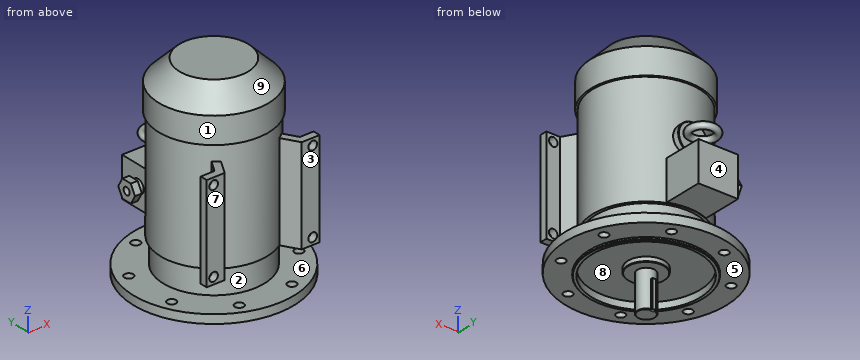
from build123d import *

# Parameters (mm, degrees)
SKETCH_1_R           = 19
EXTRUDE_1_DEPTH      = 80
SKETCH_2_W           = 8
SKETCH_2_H           = 8
EXTRUDE_2_DEPTH      = 0.1
EXTRUDE_2_DEPTH_BACK = 60
SKETCH_3_R           = 175
EXTRUDE_3_DEPTH      = 19
SKETCH_4_R           = 125
SKETCH_4_R_2         = 118
EXTRUDE_4_DEPTH      = 5
SKETCH_5_R           = 118
SKETCH_5_R_2         = 40
CUT_EXTRUDE_1_DEPTH  = 10
CHAMFER_1_SIZE       = 1
SKETCH_6_R           = 9.5
CUT_EXTRUDE_2_DEPTH  = 20
SKETCH_7_R           = 110
EXTRUDE_5_DEPTH      = 55
SKETCH_8_R           = 116
EXTRUDE_6_DEPTH      = 242
SKETCH_9_R           = 120
EXTRUDE_7_DEPTH      = 102
CHAMFER_2_SIZE       = 45
EXTRUDE_8_DEPTH      = 208
CUT_EXTRUDE_3_REACH  = 309
SKETCH_11_R          = 9.5
SKETCH_12_W          = 86
SKETCH_12_H          = 86
EXTRUDE_9_DEPTH      = 193
SKETCH_13_R          = 32
EXTRUDE_10_DEPTH     = 126
CHAMFER_3_SIZE       = 1
SKETCH_15_R          = 7
SKETCH_16_R          = 15
EXTRUDE_11_DEPTH     = 10
EXTRUDE_12_DEPTH     = 15
SKETCH_18_R          = 8
CUT_EXTRUDE_4_DEPTH  = 15


with BuildPart() as part:
    # Эскиз1 → Вытянуть1 (new body)
    with BuildSketch(Plane.XY):
        Circle(SKETCH_1_R)
    extrude(amount=EXTRUDE_1_DEPTH)

    # Эскиз2 → Вытянуть2 (add, two sides)
    with BuildSketch(Plane(origin=(0, 0, 0), x_dir=(-1, 0, 0), z_dir=(0, 0, -1))) as extrude_2_sk:
        with Locations((0, 18)):
            Rectangle(SKETCH_2_W, SKETCH_2_H)
    extrude(amount=EXTRUDE_2_DEPTH)
    extrude(extrude_2_sk.sketch, amount=-EXTRUDE_2_DEPTH_BACK)

    # Эскиз3 → Вытянуть3 (add)
    with BuildSketch(Plane.XY.offset(80)):
        Circle(SKETCH_3_R)
    extrude(amount=EXTRUDE_3_DEPTH)

    # Эскиз4 → Вытянуть4 (add)
    with BuildSketch(Plane(origin=(0, 0, 80), x_dir=(-1, 0, 0), z_dir=(0, 0, -1))):
        with Locations(Location((0, 0, 0), (0, 0, 180))):  # turned: the seam where the file's is
            Circle(SKETCH_4_R)
        Circle(SKETCH_4_R_2, mode=Mode.SUBTRACT)
    extrude(amount=EXTRUDE_4_DEPTH)

    # Эскиз5 → Вырез-Вытянуть1 (cut)
    with BuildSketch(Plane(origin=(0, 0, 80), x_dir=(-1, 0, 0), z_dir=(0, 0, -1))):
        Circle(SKETCH_5_R)
        Circle(SKETCH_5_R_2, mode=Mode.SUBTRACT)
    extrude(amount=-CUT_EXTRUDE_1_DEPTH, mode=Mode.SUBTRACT)

    # Фаска1
    chamfer_1_edges = [part.edges().sort_by_distance(p)[0] for p in [
        (-125, 0, 75),
        (40, 0, 80),
        (-11.937336386, -14.781745499, 0),
    ]]
    chamfer(chamfer_1_edges, length=CHAMFER_1_SIZE)

    # Эскиз6 → Вырез-Вытянуть2 (cut, through all)
    with BuildSketch(Plane(origin=(0, 0, 80), x_dir=(-1, 0, 0), z_dir=(0, 0, -1))):
        with Locations((-57.402514855, 138.581929877)):
            Circle(SKETCH_6_R)
        with Locations((57.402514855, 138.581929877)):
            Circle(SKETCH_6_R)
        with Locations((138.581929877, 57.402514855)):
            Circle(SKETCH_6_R)
        with Locations((138.581929877, -57.402514855)):
            Circle(SKETCH_6_R)
        with Locations((57.402514855, -138.581929877)):
            Circle(SKETCH_6_R)
        with Locations((-57.402514855, -138.581929877)):
            Circle(SKETCH_6_R)
        with Locations((-138.581929877, -57.402514855)):
            Circle(SKETCH_6_R)
        with Locations((-138.581929877, 57.402514855)):
            Circle(SKETCH_6_R)
    extrude(amount=-CUT_EXTRUDE_2_DEPTH, mode=Mode.SUBTRACT)

    # Эскиз7 → Вытянуть5 (add)
    with BuildSketch(Plane.XY.offset(99)):
        Circle(SKETCH_7_R)
    extrude(amount=EXTRUDE_5_DEPTH)

    # Эскиз8 → Вытянуть6 (add)
    with BuildSketch(Plane.XY.offset(154)):
        Circle(SKETCH_8_R)
    extrude(amount=EXTRUDE_6_DEPTH)

    # Эскиз9 → Вытянуть7 (add)
    with BuildSketch(Plane.XY.offset(396)):
        Circle(SKETCH_9_R)
    extrude(amount=EXTRUDE_7_DEPTH)

    # Фаска2
    chamfer_2_edges = [part.edges().sort_by_distance(p)[0] for p in [
        (-120, 0, 498),
    ]]
    chamfer(chamfer_2_edges, length=CHAMFER_2_SIZE)

    # Эскиз10 → Вытянуть8 (add)
    with BuildSketch(Plane(origin=(0, 0, 154), x_dir=(-1, 0, 0), z_dir=(0, 0, -1))):
        Polygon((-123, -132), (-83.762395693, -132), (-58.16412012, -87.662486121), (-72.020526581, -79.662486121), (-93, -116), (-123, -116), align=None)
        Polygon((123, -132), (83.762395693, -132), (58.16412012, -87.662486121), (72.020526581, -79.662486121), (93, -116), (123, -116), align=None)
    extrude(amount=-EXTRUDE_8_DEPTH)

    # Эскиз11 → Вырез-Вытянуть3 (cut, up to next)
    with BuildSketch(Plane.XZ.offset(132), mode=Mode.PRIVATE) as cut_extrude_3_sk1:
        with Locations((-108, 169)):
            Circle(SKETCH_11_R)
    cut_extrude_3_tool1 = extrude(cut_extrude_3_sk1.sketch, amount=-CUT_EXTRUDE_3_REACH, mode=Mode.PRIVATE) & part.part
    add(cut_extrude_3_tool1.solids().sort_by_distance((-108, -132, 169))[0], mode=Mode.SUBTRACT)
    # Эскиз11 → Вырез-Вытянуть3 (cut, up to next)
    with BuildSketch(Plane.XZ.offset(132), mode=Mode.PRIVATE) as cut_extrude_3_sk2:
        with Locations((108, 169)):
            Circle(SKETCH_11_R)
    cut_extrude_3_tool2 = extrude(cut_extrude_3_sk2.sketch, amount=-CUT_EXTRUDE_3_REACH, mode=Mode.PRIVATE) & part.part
    add(cut_extrude_3_tool2.solids().sort_by_distance((108, -132, 169))[0], mode=Mode.SUBTRACT)
    # Эскиз11 → Вырез-Вытянуть3 (cut, up to next)
    with BuildSketch(Plane.XZ.offset(132), mode=Mode.PRIVATE) as cut_extrude_3_sk3:
        with Locations((-108, 347)):
            Circle(SKETCH_11_R)
    cut_extrude_3_tool3 = extrude(cut_extrude_3_sk3.sketch, amount=-CUT_EXTRUDE_3_REACH, mode=Mode.PRIVATE) & part.part
    add(cut_extrude_3_tool3.solids().sort_by_distance((-108, -132, 347))[0], mode=Mode.SUBTRACT)
    # Эскиз11 → Вырез-Вытянуть3 (cut, up to next)
    with BuildSketch(Plane.XZ.offset(132), mode=Mode.PRIVATE) as cut_extrude_3_sk4:
        with Locations((108, 347)):
            Circle(SKETCH_11_R)
    cut_extrude_3_tool4 = extrude(cut_extrude_3_sk4.sketch, amount=-CUT_EXTRUDE_3_REACH, mode=Mode.PRIVATE) & part.part
    add(cut_extrude_3_tool4.solids().sort_by_distance((108, -132, 347))[0], mode=Mode.SUBTRACT)

    # Эскиз12 → Вытянуть9 (add)
    with BuildSketch(Plane(origin=(0, 0, 0), x_dir=(1, 0, 0), z_dir=(0, 1, 0))):
        with Locations((0, -198)):
            Rectangle(SKETCH_12_W, SKETCH_12_H)
    extrude(amount=EXTRUDE_9_DEPTH)

    # Эскиз13 → Вытянуть10 (add)
    with BuildSketch(Plane(origin=(0, 0, 0), x_dir=(1, 0, 0), z_dir=(0, 1, 0))):
        with Locations(Location((0, -286, 0), (0, 0, 90))):  # turned: the seam where the file's is
            Circle(SKETCH_13_R)
    extrude(amount=EXTRUDE_10_DEPTH)

    # Фаска3
    chamfer_3_edges = [part.edges().sort_by_distance(p)[0] for p in [
        (0, 126, 318),
    ]]
    chamfer(chamfer_3_edges, length=CHAMFER_3_SIZE)

    # По траектории1: sweep along a path in Эскиз14
    with BuildLine(Plane.XY.offset(286)) as sweep_1_path:
        CenterArc((0, 152), 26, 0, 360)
    # Эскиз15 → По траектории1 (sweep)
    with BuildSketch(Plane(origin=(0, 0, 0), x_dir=(0, 0, -1), z_dir=(1, 0, 0))):
        with Locations((-286, 178)):
            Circle(SKETCH_15_R)
    sweep(path=sweep_1_path.line)

    # Эскиз16 → Вытянуть11 (add)
    with BuildSketch(Plane.ZY.offset(43)):
        with Locations(Location((198, 150, 0), (0, 0, 180))):  # turned: the seam where the file's is
            Circle(SKETCH_16_R)
    extrude(amount=EXTRUDE_11_DEPTH)

    # Эскиз17 → Вытянуть12 (add)
    with BuildSketch(Plane.ZY.offset(53)):
        Polygon((198, 172.516660498), (178.5, 161.258330249), (178.5, 138.741669751), (198, 127.483339502), (217.5, 138.741669751), (217.5, 161.258330249), align=None)
    extrude(amount=EXTRUDE_12_DEPTH)

    # Эскиз18 → Вырез-Вытянуть4 (cut)
    with BuildSketch(Plane.ZY.offset(68)):
        with Locations((198, 150)):
            Circle(SKETCH_18_R)
    extrude(amount=-CUT_EXTRUDE_4_DEPTH, mode=Mode.SUBTRACT)


solid = part.part
Geometry check sheet. Reference: the model listing, model coordinates, mm. Face numbers are marked on the shaded views. A direction names the side the tool comes from. Coordinates: 2 decimals unless noted, no trailing zeros. Order: outer loops, then holes, each group sorted by start corner. A loop starts at its lowest first (then second) coordinate and runs counter-clockwise, first axis right, second up. Notation, with made-up numbers: (59, 1.25) - (74, 1.25) arc R23 ccw to (74, 39.25) - close; hole circle Ø4 at (4.25, -26.75). An arc over 180 degrees is marked (long way). Answer in a Markdown table with one row per item. Add a question column.
1) Release check for a two-part mould opening along Z. For the marked faces 6, 7, 8 and 9 record: +Z half, -Z half, draft (parallel to the pull), parting line (faces both ways), or undercut.
2) Cross-section at A-A, the plane z = 347. Record the cut outline in (x, y).
3) Gauge pin test, flat ends, axial feed: P1, Ø9, axis at y = 18.5, z = 37, coming from the -X side; P2, Ø22, axis at x = 108, z = 169, coming from the +Y side; P3, Ø10, axis at x = 95.5, z = 407, coming from the -Y side; P4, Ø12, axis at x = -74.5, y = 26, coming from the +Z side. Record the tip position at first contact, or that the pin passes through.
4) Set-up check for the marked faces 1, 2, 3, 4 and 5: record each of +Z, -Z, +X, -X, +Y, -Y from which the full face is reachable in a straight line by a thin tool's end or side.
5) Material ranges on line 1 along Z through (x, y) = (108, -127.25); line 2 along Y through (x, z) = (-62.5, 198); line 3 along Z through (x, y) = (36, 157), recorded low to high. Write a range as [from, to].
6) Cross-section at C-C, the plane z = 107. Record the cut outline in (x, y).
7) Cross-section at B-B, the plane z = 286. Record the cut outline in (x, y), then the cut area to 3 significant figures.
8) Cross-section at D-D, the plane z = 169. Record the cut outline in (x, y).
Check result:
| question | item | result |
|---|---|---|
| 1 | face 6 | undercut |
| 1 | face 7 | draft |
| 1 | face 8 | -Z half |
| 1 | face 9 | +Z half |
| 2 | outline | (-123, -132) - (-117.5, -132) - (-117.5, -116) - (-123, -116) - close; (-98.5, -132) - (-83.76, -132) - (-63.57, -97.03) arc R116 ccw to (63.57, -97.03) - (83.76, -132) - (98.5, -132) - (98.5, -116) - (93, -116) - (76.42, -87.27) arc R116 ccw (long way) to (-76.42, -87.27) - (-93, -116) - (-98.5, -116) - close; (117.5, -132) - (123, -132) - (123, -116) - (117.5, -116) - close |
| 3 | P1 | stops at x = -12.85 |
| 3 | P2 | stops at y = 63.62 |
| 3 | P3 | stops at y = -78.8 |
| 3 | P4 | stops at z = 498 |
| 4 | face 1 | +Z |
| 4 | face 2 | none |
| 4 | face 3 | +Z, +X, -X, -Y |
| 4 | face 4 | +Z, -Z, +X, -X, +Y |
| 4 | face 5 | -Z |
| 5 | line 1 | z = [80, 99], [154, 159.5], [178.5, 337.5], [356.5, 362] |
| 5 | line 2 | y = [-97.72, 97.72], [127.48, 142], [158, 172.52] |
| 5 | line 3 | z = [80, 99], [155, 241] |
| 6 | outline | circle Ø220 at (0, 0) |
| 7 | outline | (-123, -132) - (-83.76, -132) - (-63.57, -97.03) arc R116 ccw to (63.57, -97.03) - (83.76, -132) - (123, -132) - (123, -116) - (93, -116) - (76.42, -87.27) arc R116 ccw to (32, 111.5) - (32, 125) - (31, 126) - (20.32, 126) arc R33 ccw (long way) to (-20.32, 126) - (-31, 126) - (-32, 125) - (-32, 111.5) arc R116 ccw to (-76.42, -87.27) - (-93, -116) - (-123, -116) - close; hole circle Ø38 at (0, 152) |
| 7 | area | 47,400 mm² |
| 8 | outline | (-123, -132) - (-117.5, -132) - (-117.5, -116) - (-123, -116) - close; (-98.5, -132) - (-83.76, -132) - (-63.57, -97.03) arc R116 ccw to (63.57, -97.03) - (83.76, -132) - (98.5, -132) - (98.5, -116) - (93, -116) - (76.42, -87.27) arc R116 ccw to (43, 107.74) - (43, 193) - (-43, 193) - (-43, 107.74) arc R116 ccw to (-76.42, -87.27) - (-93, -116) - (-98.5, -116) - close; (117.5, -132) - (123, -132) - (123, -116) - (117.5, -116) - close |
